Source: CAD feature listing. Evaluate the final solid. Frame: model axes, mm. Coordinates: 2 decimals unless noted, no trailing zeros. Write each loop counter-clockwise with the first axis right and the second up, starting at its lowest first coordinate (ties: lowest second). Pieces come first, ordered by that corner, then holes. Notation, with made-up numbers: (72.5, 18) - (126.5, 18) arc R16 ccw to (126.5, 42) - close; hole circle Ø7 at (70, -24.5). An arc over 180 degrees is marked (long way). One line per item, written item: value.
from build123d import *

# Parameters (mm, degrees)
BOSS_EXTRU_1_DEPTH = 9
CONG_1_R           = 1000
CONG_2_R           = 250
CONG_4_R           = 10
CONG_5_R           = 5
CONG_6_R           = 100


with BuildPart() as part:
    # Esquisse2 → Boss.-Extru.1 (new body)
    with BuildSketch(Plane.XY):
        Polygon((0, 0), (-753.514541491, 0), (-915.190229508, 170.50346618), (-1093.283519558, 392.387219436), (-1007.982904338, 368.608976512), (-1007.982904338, 347.108976512), (-1004.982904338, 347.108976512), (-1004.982904338, 366.343498655), (-875.399006988, 219.616732713), (-811.570765603, 152.303356597), (-811.570765603, 130.803356597), (-808.570765603, 130.803356597), (-808.570765603, 150.375814407), (-755.274625166, 94.639899826), (-627.232048759, 94.639899826), (-627.232048759, 73.139899826), (-624.232048759, 73.139899826), (-624.232048759, 94.639899826), (-242.444799847, 94.639899826), (-242.444799847, 73.139899826), (-239.444799847, 73.139899826), (-239.444799847, 94.639899826), (-218.449092799, 94.639899826), (-46.093252688, 403.139899826), (-12.434439882, 403.139899826), (-12.434439882, 253.139899826), (-9.434439882, 253.139899826), (-9.434439882, 136.779854294), (-82.801847324, 99.620582608), (-82.801847324, 26.059273195), (0, 25.118109707), align=None)
    extrude(amount=BOSS_EXTRU_1_DEPTH)

    # Congé1
    # the kernel refuses this fillet: 1000 mm, written as the material it takes off along each edge
    with BuildSketch(Plane(origin=(-915.190229508, 170.50346618, -103.157271439), x_dir=(0.6880722367162745, -0.7256421963063223, 0), z_dir=(0, 0, 1))) as cong_1_piece_1:
        with BuildLine():
            CenterArc((CONG_1_R * 0.0412629085755, CONG_1_R), CONG_1_R, 265.274299796, 4.725700204)
            Line((-CONG_1_R * 0.0411226366703, CONG_1_R * 0.00339946722142), (0, 0))
            Line((0, 0), (CONG_1_R * 0.0412629085755, 0))
        make_face()
    extrude(amount=215.314542878, mode=Mode.SUBTRACT)

    # Congé2
    cong_2_edges = [part.edges().sort_by_distance(p)[0] for p in [
        (-753.514541491, 0, 4.5),
    ]]
    fillet(cong_2_edges, radius=CONG_2_R)

    # Congé4
    cong_4_edges = [part.edges().sort_by_distance(p)[0] for p in [
        (0, 0, 4.5),
    ]]
    fillet(cong_4_edges, radius=CONG_4_R)

    # Congé5
    cong_5_edges = [part.edges().sort_by_distance(p)[0] for p in [
        (-1093.283519558, 392.387219436, 4.5),
    ]]
    fillet(cong_5_edges, radius=CONG_5_R)

    # Congé6
    cong_6_edges = [part.edges().sort_by_distance(p)[0] for p in [
        (-755.274625166, 94.639899826, 4.5),
    ]]
    fillet(cong_6_edges, radius=CONG_6_R)


solid = part.part
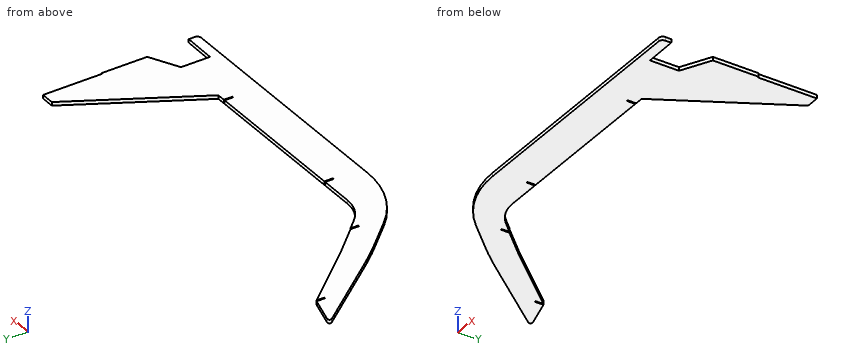
1) Material intervals for line 1 (X direction, y = 360, z = 6); line 2 (Y direction, x = -449.5, z = 4); line 3 (X direction, y = 363, z = 6.25), sorted ascending.
Values found:
line 1: -1067.29 to -1007.98, -1004.98 to -999.38, -70.2 to -12.43
line 2: 0 to 94.64
line 3: -1069.7 to -1007.98, -1004.98 to -1002.03, -68.52 to -12.43
2) Section query A-A on y = 298.5. Output: boundary loops of the cut face in (x, z).
Values found:
outline: (-1017.93, 0) - (-945.07, 0) - (-945.07, 9) - (-1017.93, 9) - close; (-104.55, 0) - (-12.43, 0) - (-12.43, 9) - (-104.55, 9) - close
3) Section query C-C on y = 46.5. Output: boundary loops of the cut face in (x, z).
Values found:
outline: (-791.26, 0) - (-82.8, 0) - (-82.8, 9) - (-791.26, 9) - close
4) Section query B-B on x = -355. Output: boundary loops of the cut face in (y, z), then the cut area to 3 significant figures.
Values found:
outline: (0, 0) - (94.64, 0) - (94.64, 9) - (0, 9) - close
area: 852 mm2
5) Contact query for flat-ended pins moving along their axis: P1, Ø4.5, axis at x = -230.5, z = 6, coming from the +Y side; P2, Ø3, axis at y = 131.5, z = 2, coming from the +X side; P3, Ø4.5, axis at y = 84, z = 3, coming from the -X side. Output: stop coordinate, or through.
Values found:
P1: y = 94.64
P2: x = -16.9
P3: x = -835.3
